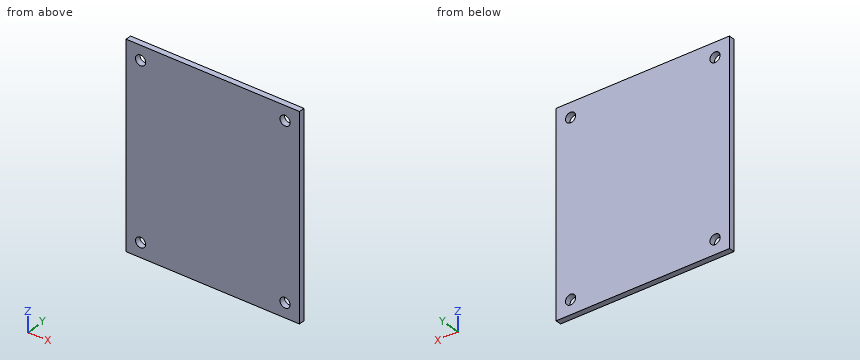
Autodesk Inventor part; units mm, degrees
ref_plane "YZ Plane" through (0, 0, 0) normal (1, 0, 0) x (0, 1, 0)
ref_plane "XZ Plane" through (0, 0, 0) normal (0, 1, 0) x (-1, 0, 0)
ref_plane "XY Plane" through (0, 0, 0) normal (0, 0, 1) x (1, 0, 0)
sketch "Sketch1" plane through (0, 0, 0) normal (0, 1, 0) x (-1, 0, 0)
  line L0 (30, 48.6275) -> (-30, 48.6275)
  line L1 (-30, 48.6275) -> (-30, -21.3725)
  line L2 (-30, -21.3725) -> (30, -21.3725)
  line L3 (30, -21.3725) -> (30, 48.6275)
  point P0 (0, 0)
  dimension "d0" = 70
  dimension "d1" = 60
extrude "Extrusion1" add sketch "Sketch1" along normal blind 2
sketch "Sketch2" plane through (0, 2, 0) normal (0, 1, 0) x (1, 0, 0)
  line L0 (0, 0) -> (-21.5262, 0) construction
  circle A0 centre (-25, -43.6275) radius 1.75
  line L1 (-30, -48.6275) -> (30, -48.6275)
  line L2 (-30, 21.3725) -> (-30, -48.6275)
  circle A1 centre (25, -43.6275) radius 1.75
  circle A2 centre (25, 16.3725) radius 1.75
  circle A3 centre (-25, 16.3725) radius 1.75
  line L3 (30, -48.6275) -> (30, 21.3725)
  line L4 (30, 21.3725) -> (-30, 21.3725)
  dimension "d4" = 3.5
  dimension "d5" = 5
  dimension "d6" = 5
  dimension "d7" = 3.5
  dimension "d8" = 3.5
  dimension "d9" = 3.5
  dimension "d10" = 5
  dimension "d11" = 5
  dimension "d12" = 5
  dimension "d13" = 5
  dimension "d14" = 5
  dimension "d15" = 5
extrude "Extrusion2" cut sketch "Sketch2" against normal through all contours A0 | A1 | A2 | A3
properties part number "Supporto1"
Can you work these out from the model? Positions are in its coordinate system, mm. Give positions to 0.01 mm unless a question says otherwise; leave off trailing zeros. Loops run counter-clockwise (first coordinate to the right, second up) from the corner with the lowest first, then second, coordinate; pieces in that order, holes last. Notation, with made-up numbers: M -14.75,32 L -7.75,32 A34 cw -7.75,64 Z; hole C 84,29 d8. An arc over 180 degrees is marked long. One line per item, written item: value.
1) I'm going to push a flat-ended pin straight in: pin 1 (3 mm diameter, centred on x = -25, z = 43.63, fed in from +Y). Where does the tip first touch, or does it pass through?
Geometry check:
pin 1: passes through
2) Imagine slicing it at A-A on x = -25. Write out the boundary of the cut face in (y, z), and give its area (3 significant figures).
Geometry check:
outline: M 0,-21.37 L 2,-21.37 L 2,-18.12 L 0,-18.12 Z; M 0,-14.62 L 2,-14.62 L 2,41.88 L 0,41.88 Z; M 0,45.38 L 2,45.38 L 2,48.63 L 0,48.63 Z
area: 126 mm²
3) Please list where these lines run through material, in increasing order: line 1 (Z direction, x = -25, y = 0.8); line 2 (Z direction, x = -25.5, y = 0.2).
Geometry check:
line 1: z = -21.37 to -18.12, -14.62 to 41.88, 45.38 to 48.63
line 2: z = -21.37 to -18.05, -14.7 to 41.95, 45.3 to 48.63
